For this review, take the finished solid that the model builds, in its own axes (mm). A direction names the side the tool comes from. Round coordinates to 2 decimals unless told otherwise and drop trailing zeros. Order: outer loops, then holes, each group sorted by start corner. A loop starts at its lowest first (then second) coordinate and runs counter-clockwise, first axis right, second up. Notation, with made-up numbers: (68.5, -5) -> (78.5, -5) arc R20 cw to (78.5, 28) -> close; hole circle Ø1 at (33.5, -20). An arc over 180 degrees is marked (long way). Use a Markdown table: item, result. Add a question column.
1) Consider section A-A (z = 4). Give the number of separate pieces and of enclosed holes in the cut face, plus the area to 3 significant figures.
2) Machinability: for faces 5 (the face through (17.93, 14.04, 2.95)), 6 (the face through (17.393, -13, 4)), 7 (the face through (-26, -3, 3)), 8 (the face through (17, 4, 4)), 9 (the face through (13.2, -6.79, 2.94)), which of the approach directions +Z, -Z, +X, -X, +Y, -Y give a long, thin tool a straight path to every point of the face, cutting with its end or side? Answer none if there is none.
3) Clearance check with flat-ended pins moving along their axes: P1, Ø3.5, axis at y = -13, z = 3, coming from the -X side; P2, Ø1, axis at y = 10, z = 10, coming from the +X side; P3, Ø1.5, axis at y = 0, z = 11, coming from the +X side; P4, Ø6, axis at y = -7.5, z = 9.5, coming from the -X side. State where each tip first meets the part, or that it passes through.
4) Consider section B-B (y = 0). State the section outline as (x, z) points, plus the area to 3 significant figures.
5) Draft analysis for pull direction Y (two halves, no side actions). For faces 1 (the face through (13.2, 7.7, 2.94)), 2 (the face through (15, 11.5, 2)), 3 (the face through (-12.65, -0.5, 0.84)), 4 (the face through (-12.49, -0.49, 4.45)), state which applies: pulls with the +Y half, pulls with the -Y half, needs draft (parallel to the pull), parting line crosses it, or undercut.
6) Consider section D-D (z = 17.75). State the section outline as (x, y) points.
7) Wall thickness on line 1 along X through (y, z) = (0, 11.25); line 2 along Y through (x, z) = (-29.5, 12.5); line 3 along Y through (x, z) = (18, 2): over which ranges is each line inside the solid? List them lowest first. Write a range as [from, to].
8) Consider section C-C (x = 0). State the section outline as (y, z) points.
```python
from build123d import *

# Parameters (mm, degrees)
ESBO_O1_R                = 4
RESSALTO_EXTRUS_O1_DEPTH = 20
ESBO_O2_OUTSIDE_W        = 75.1
ESBO_O2_OUTSIDE_H        = 49.1
ESBO_O2_OUTSIDE_R        = 9
CORTE_EXTRUS_O1_DEPTH    = 12
FILETE1_R                = 55
ESBO_O3_R                = 5.15
CORTE_EXTRUS_O2_DEPTH    = 3
CORTE_EXTRUS_O3_START    = -20
ESBO_O3_2_R              = 5.15
CORTE_EXTRUS_O3_DEPTH    = 3
ESBO_O4_R                = 1.75
CORTE_EXTRUS_O4_DEPTH    = 34
CORTE_EXTRUS_O5_DEPTH    = 7
ESBO_O6_R                = 3.5
CORTE_EXTRUS_O6_DEPTH    = 5
CHANFRO1_SIZE            = 1


with BuildPart() as part:
    # Esboço1 → Ressalto-extrusão1 (new body)
    with BuildSketch(Plane.XY):
        with BuildLine():
            Line((-20.5, 16.5), (-34.372611465, 7.566878981))
            ThreePointArc((-34.372611465, 7.566878981), (-38.5, 0), (-34.372611465, -7.566878981))
            Line((-34.372611465, -7.566878981), (-20.5, -16.5))
            Line((-20.5, -16.5), (20.5, -16.5))
            Line((20.5, -16.5), (20.5, -4))
            Line((20.5, -4), (11.842719282, -4))
            ThreePointArc((11.842719282, -4), (-12.5, 0), (11.842719282, 4))
            Line((11.842719282, 4), (20.5, 4))
            Line((20.5, 4), (20.5, 16.5))
            Line((20.5, 16.5), (-20.5, 16.5))
        make_face()
        with Locations((-29.5, 0)):
            Circle(ESBO_O1_R, mode=Mode.SUBTRACT)
    extrude(amount=RESSALTO_EXTRUS_O1_DEPTH)

    # Esboço2 outside → Corte-extrusão1 (cut)
    with BuildSketch(Plane.XY.offset(20)):
        with Locations((-9, 0)):
            Rectangle(ESBO_O2_OUTSIDE_W, ESBO_O2_OUTSIDE_H)
        with Locations((-29.5, 0)):
            Circle(ESBO_O2_OUTSIDE_R, mode=Mode.SUBTRACT)
    extrude(amount=-CORTE_EXTRUS_O1_DEPTH, mode=Mode.SUBTRACT)

    # Filete1
    filete1_edges = [part.edges().sort_by_distance(p)[0] for p in [
        (-20.5, -16.5, 4),
        (-20.5, 16.5, 4),
    ]]
    fillet(filete1_edges, radius=FILETE1_R)

    # Esboço3 → Corte-extrusão2 (cut)
    with BuildSketch(Plane.XY.offset(20)):
        with Locations((-29.5, 0)):
            Circle(ESBO_O3_R)
    extrude(amount=-CORTE_EXTRUS_O2_DEPTH, mode=Mode.SUBTRACT)

    # Esboço3<2> → Corte-extrusão3 (cut)
    with BuildSketch(Plane.XY.offset(20).offset(CORTE_EXTRUS_O3_START)):
        with Locations((-29.5, 0)):
            Circle(ESBO_O3_2_R)
    extrude(amount=CORTE_EXTRUS_O3_DEPTH, mode=Mode.SUBTRACT)

    # Esboço4 → Corte-extrusão4 (cut, through all)
    with BuildSketch(Plane.XZ.offset(16.5)):
        with Locations((14.592719282, 4)):
            Circle(ESBO_O4_R)
    extrude(amount=-CORTE_EXTRUS_O4_DEPTH, mode=Mode.SUBTRACT)

    # Esboço5 → Corte-extrusão5 (cut)
    with BuildSketch(Plane.XZ.offset(16.5)):
        Polygon((14.592719282, 7.233161507), (11.792719282, 5.616580754), (11.792719282, 2.383419246), (14.592719282, 0.766838493), (17.392719282, 2.383419246), (17.392719282, 5.616580754), align=None)
    extrude(amount=-CORTE_EXTRUS_O5_DEPTH, mode=Mode.SUBTRACT)

    # Esboço6 → Corte-extrusão6 (cut)
    with BuildSketch(Plane(origin=(0, 16.5, 0), x_dir=(1, 0, 0), z_dir=(0, 1, 0))):
        with Locations((14.592719282, -4)):
            Circle(ESBO_O6_R)
    extrude(amount=-CORTE_EXTRUS_O6_DEPTH, mode=Mode.SUBTRACT)

    # Chanfro1
    chanfro1_edges = [part.edges().sort_by_distance(p)[0] for p in [
        (-12.5, 0, 0),
        (-34.65, 0, 0),
    ]]
    chamfer(chanfro1_edges, length=CHANFRO1_SIZE)


solid = part.part
```
Results list:
| question | item | result |
|---|---|---|
| 1 | separate pieces | 3 |
| 1 | enclosed holes | 1 |
| 1 | area | 956 mm2 |
| 2 | face 5 | +Y |
| 2 | face 6 | -Y |
| 2 | face 7 | -Z |
| 2 | face 8 | +Z, -Z, +X |
| 2 | face 9 | +Y, -Y |
| 3 | P1 | x = -27.77 |
| 3 | P2 | through |
| 3 | P3 | x = -20.5 |
| 3 | P4 | x = -37.29 |
| 4 | outline | (-38.5, 0) -> (-35.65, 0) -> (-34.65, 1) -> (-34.65, 3) -> (-33.5, 3) -> (-33.5, 17) -> (-34.65, 17) -> (-34.65, 20) -> (-38.5, 20) -> close; (-25.5, 3) -> (-24.35, 3) -> (-24.35, 1) -> (-23.35, 0) -> (-13.5, 0) -> (-12.5, 1) -> (-12.5, 8) -> (-20.5, 8) -> (-20.5, 20) -> (-24.35, 20) -> (-24.35, 17) -> (-25.5, 17) -> close |
| 4 | area | 249 mm2 |
| 5 | face 1 | needs draft |
| 5 | face 2 | pulls with the +Y half |
| 5 | face 3 | undercut |
| 5 | face 4 | undercut |
| 6 | outline | circle Ø18 at (-29.5, 0); hole circle Ø10.3 at (-29.5, 0) |
| 7 | line 1 | [-38.5, -33.5], [-25.5, -20.5] |
| 7 | line 2 | [-9, -4], [4, 9] |
| 7 | line 3 | [-16.5, -4], [4, 16.5] |
| 8 | outline | (-16.5, 0) -> (-13.5, 0) -> (-12.5, 1) -> (-12.5, 8) -> (-16.5, 8) -> close; (12.5, 1) -> (13.5, 0) -> (16.5, 0) -> (16.5, 8) -> (12.5, 8) -> close |
